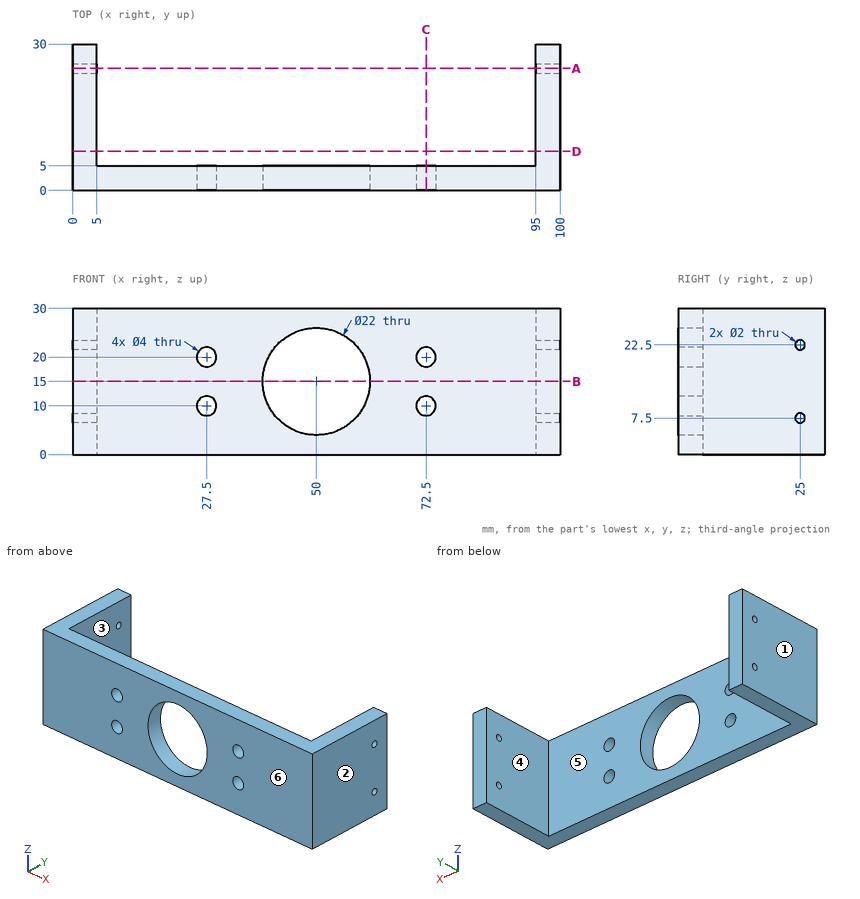
Print and shaded views of the part. All mm, measured from the part's lowest x, y and z. A direction names the side the tool comes from. Coordinates: 2 decimals unless noted, no trailing zeros. Write each loop counter-clockwise with the first axis right and the second up, starting at its lowest first coordinate (ties: lowest second). Pieces come first, ordered by that corner, then holes.
(1) Cut at B-B, the plane z = 15. List the corners of the cut face in (x, y), and give its area (3 significant figures).
(2) Cut at D-D, the plane y = 8. List the corners of the cut face in (x, z).
(3) 3-axis set-ups, long thin cutter, end or side, ignore diameter. For the marked faces 5 and 6: which of +Z, -Z, +X, -X, +Y, -Y reach the whole face in a straight line?
(4) Cut at C-C, the plane x = 72.5. List the corners of the cut face in (y, z), and give its area (3 significant figures).
(5) Flat gauge pins, fed straight in: pin 1 (12 mm diameter, centred on y = 21, z = 7.5, fed in from -X); pin 2 (6.5 mm diameter, centred on x = 27.5, z = 10, fed in from +Y); pin 3 (3.5 mm diameter, centred on x = 27.5, z = 20, fed in from -Y). Where does each tip first touch, or does it go through?
(6) Drill centre lines: probe 1 along X at (y, z) = (12, 21.5); probe 2 along Y at (x, z) = (96.1, 7.5); probe 3 along Y at (x, z) = (14, 15.5). Where is each one in solid material? Low to high.
(7) Two-plate mould, pull along X, no slides. Class the marked faces 1, 2, 3 and 4: +X half, -X half, draft (parallel to the pull), parting line (faces both ways), or undercut.
(8) Cut at A-A, the plane y = 25. List the corners of the cut face in (x, z), and give its area (3 significant figures).
Geometry says:
1. outline: (0, 0) - (39, 0) - (39, 5) - (5, 5) - (5, 30) - (0, 30) - close; (61, 0) - (100, 0) - (100, 30) - (95, 30) - (95, 5) - (61, 5) - close
1. area: 640 mm2
2. outline: (0, 0) - (5, 0) - (5, 30) - (0, 30) - close; (95, 0) - (100, 0) - (100, 30) - (95, 30) - close
3. face 5: +Z, -Z, +Y
3. face 6: +Z, -Z, +X, -X, -Y
4. outline: (0, 0) - (5, 0) - (5, 8) - (0, 8) - close; (0, 12) - (5, 12) - (5, 18) - (0, 18) - close; (0, 22) - (5, 22) - (5, 30) - (0, 30) - close
4. area: 110 mm2
5. pin 1: stops at x = 0
5. pin 2: stops at y = 5
5. pin 3: passes through
6. probe 1: x = 0 to 5, 95 to 100
6. probe 2: y = 0 to 24, 26 to 30
6. probe 3: y = 0 to 5
7. face 1: -X half
7. face 2: +X half
7. face 3: undercut
7. face 4: undercut
8. outline: (0, 0) - (5, 0) - (5, 6.5) - (0, 6.5) - close; (0, 8.5) - (5, 8.5) - (5, 21.5) - (0, 21.5) - close; (0, 23.5) - (5, 23.5) - (5, 30) - (0, 30) - close; (95, 0) - (100, 0) - (100, 6.5) - (95, 6.5) - close; (95, 8.5) - (100, 8.5) - (100, 21.5) - (95, 21.5) - close; (95, 23.5) - (100, 23.5) - (100, 30) - (95, 30) - close
8. area: 260 mm2
